from build123d import *

# Parameters (mm, degrees)
F1_DEPTH = 20
F3_DEPTH = 3
F4_W     = 22
F4_H     = 30
F5_DEPTH = 13.8
F6_W     = 28.5
F6_H     = 2.2146213427
F7_DEPTH = 3
F8_R     = 1


with BuildPart() as f1:
    # F0 (on Top) → F1 (new body)
    with BuildSketch(Plane.XY):
        Polygon((0, 22.5), (-17.5, 22.5), (-17.5, 0), (-14.605, 0), (0, 0), (0, 20.066), align=None)
        Polygon((17.5, 22.5), (0, 22.5), (0, 20.066), (0, 0), (-14.605, 0), (-17.5, 0), (-17.5, -22.5), (17.5, -22.5), align=None)
    extrude(amount=F1_DEPTH)

    # F2 (on face) → F3 (cut)
    with BuildSketch(Plane.XY.offset(20)):
        Polygon((0.1571281302, 20.2146213427), (-14.0928718698, 20.2146213427), (-14.0928718698, 0), (-14.0928718698, -20.2853786573), (14.4071281302, -20.2853786573), (14.4071281302, 20.2146213427), align=None)
    extrude(amount=-F3_DEPTH, mode=Mode.SUBTRACT)

    # F4 (on face) → F5 (cut)
    with BuildSketch(Plane.XY.offset(17)):
        Rectangle(F4_W, F4_H)
    extrude(amount=-F5_DEPTH, mode=Mode.SUBTRACT)

    # F6 (on face) → F7 (cut, through all)
    with BuildSketch(Plane.XY.offset(20)):
        with Locations((0.1571281302, -21.3926893286)):
            Rectangle(F6_W, F6_H)
    extrude(amount=-F7_DEPTH, mode=Mode.SUBTRACT)

    # F8
    f8_edges = [f1.edges().sort_by_distance(p)[0] for p in [
        (-11, 0, 3.2),
        (0, -15, 3.2),
        (0, 15, 3.2),
        (11, 0, 3.2),
        (0, 15, 17),
        (11, 0, 17),
        (-11, 0, 17),
        (0, -15, 17),
        (11, 15, 10.1),
        (-11, 15, 10.1),
        (11, -15, 10.1),
        (-11, -15, 10.1),
    ]]
    fillet(f8_edges, radius=F8_R)


solid = f1.part
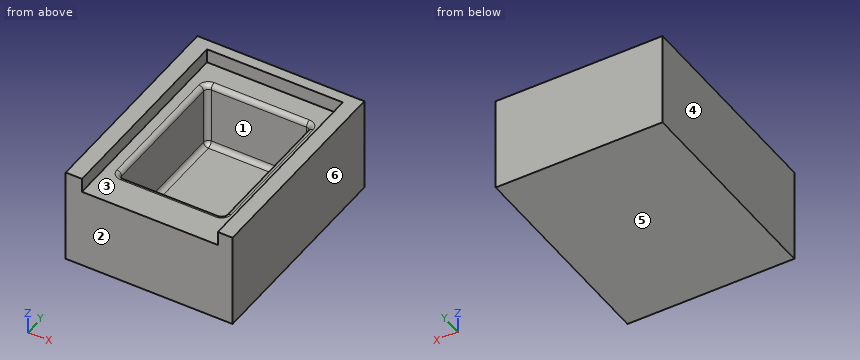
The model under review builds one solid part; all positions refer to its coordinate system, in mm. Face numbers are marked on the shaded views. A direction names the side the tool comes from. Round coordinates to 2 decimals unless told otherwise and drop trailing zeros. Loops run counter-clockwise (first coordinate to the right, second up) from the corner with the lowest first, then second, coordinate; pieces in that order, holes last. Notation, with made-up numbers: (38, 5) -> (52, 5) arc R17 cw to (52, 24) -> close; hole circle Ø7 at (84.25, -31.75). An arc over 180 degrees is marked (long way). One line per question, with ' | ' between items. Start each with the question number.
Item 1: Add section A-A, the plane z = 12.5. Write out the cut boundary in (x, y).
Item 2: Draft analysis for pull direction X (two halves, no side actions). For the marked faces 3, 4, 5 and 6, state which applies: +X half, -X half, draft (parallel to the pull), parting line (faces both ways), or undercut.
Item 3: Add section D-D, the plane y = 9. Write out the cut boundary in (x, z).
Item 4: Add section C-C, the plane x = 2. Write out the cut boundary in (y, z).
Item 5: Machinability: for the marked faces 1 and 2, which of the approach directions +Z, -Z, +X, -X, +Y, -Y give a long, thin tool a straight path to every point of the face, cutting with its end or side? Answer none if there is none.
Item 6: For pin 1 (10 mm diameter, centred on x = -7, y = 14, fed in from +Z); pin 2 (16 mm diameter, centred on x = -1.5, y = -0.5, fed in from +Z), all flat-tipped, find the tip position at first contact; note any pin that passes through.
Item 7: Add section B-B, the plane y = -18. Write out the cut boundary in (x, z).
Item 8: Wall thickness on line 1 along X through (y, z) = (7.5, 8.25); line 2 along Y through (x, z) = (7.5, 13.75); line 3 along Z through (x, y) = (4, -13.5): over which ranges is each line inside the solid? List them lowest first. Write a range as [from, to].
Return value:
1) outline: (-17.5, -22.5) -> (17.5, -22.5) -> (17.5, 22.5) -> (-17.5, 22.5) -> close; hole (-11, -14) arc R1 ccw to (-10, -15) -> (10, -15) arc R1 ccw to (11, -14) -> (11, 14) arc R1 ccw to (10, 15) -> (-10, 15) arc R1 ccw to (-11, 14) -> close
2) face 3: undercut | face 4: -X half | face 5: draft | face 6: +X half
3) outline: (-17.5, 0) -> (17.5, 0) -> (17.5, 20) -> (14.41, 20) -> (14.41, 17) -> (12, 17) arc R1 ccw to (11, 16) -> (11, 4.2) arc R1 cw to (10, 3.2) -> (-10, 3.2) arc R1 cw to (-11, 4.2) -> (-11, 16) arc R1 ccw to (-12, 17) -> (-14.09, 17) -> (-14.09, 20) -> (-17.5, 20) -> close
4) outline: (-22.5, 0) -> (22.5, 0) -> (22.5, 20) -> (20.21, 20) -> (20.21, 17) -> (16, 17) arc R1 ccw to (15, 16) -> (15, 4.2) arc R1 cw to (14, 3.2) -> (-14, 3.2) arc R1 cw to (-15, 4.2) -> (-15, 16) arc R1 ccw to (-16, 17) -> (-22.5, 17) -> close
5) face 1: +Z | face 2: +Z, -Z, +X, -X, -Y
6) pin 1: stops at z = 17 | pin 2: stops at z = 3.2
7) outline: (-17.5, 0) -> (17.5, 0) -> (17.5, 20) -> (14.41, 20) -> (14.41, 17) -> (-14.09, 17) -> (-14.09, 20) -> (-17.5, 20) -> close
8) line 1: x = [-17.5, -11], [11, 17.5] | line 2: y = [-22.5, -15], [15, 22.5] | line 3: z = [0, 3.2]
